from build123d import *

# Parameters (mm, degrees)
SKETCH_1_R               = 5
EXTRUDE_1_DEPTH          = 10
SKETCH_3_R               = 25
SKETCH_3_R_2             = 5
EXTRUDE_4_DEPTH          = 10
EXTRUDE_5_REACH          = 111.952
SKETCH_11_R              = 25
CUT_EXTRUDE_5_DEPTH      = 110.952122557
CUT_EXTRUDE_5_DEPTH_BACK = 110.952122557
SKETCH_13_R              = 18
RIB_2_REACH              = 111.126
SKETCH_14_WALL_W         = 252.93163968
SKETCH_14_WALL_H         = 10
CUT_EXTRUDE_6_DEPTH      = 110.126073878
CUT_EXTRUDE_6_DEPTH_BACK = 5
RIB_3_REACH              = 119.31
SKETCH_18_WALL_W         = 268.526863554
SKETCH_18_WALL_H         = 10


with BuildPart() as part:
    # 草图1 → 凸台-拉伸1 (new body)
    with BuildSketch(Plane(origin=(0, 0, 0), x_dir=(1, 0, 0), z_dir=(0, 1, 0))):
        with BuildLine():
            Line((-50.5, 37.5), (50.5, 37.5))
            ThreePointArc((50.5, 37.5), (58.985281374, 33.985281374), (62.5, 25.5))
            Line((62.5, 25.5), (62.5, -25.5))
            ThreePointArc((62.5, -25.5), (58.985281374, -33.985281374), (50.5, -37.5))
            Line((50.5, -37.5), (-50.5, -37.5))
            ThreePointArc((-50.5, -37.5), (-58.985281374, -33.985281374), (-62.5, -25.5))
            Line((-62.5, -25.5), (-62.5, 25.5))
            ThreePointArc((-62.5, 25.5), (-58.985281374, 33.985281374), (-50.5, 37.5))
        make_face()
        with Locations(Location((50.5, -25.5, 0), (0, 0, 270))):
            Circle(SKETCH_1_R, mode=Mode.SUBTRACT)
        with Locations(Location((50.5, 25.5, 0), (0, 0, 270))):
            Circle(SKETCH_1_R, mode=Mode.SUBTRACT)
        with Locations(Location((-50.5, 25.5, 0), (0, 0, 270))):
            Circle(SKETCH_1_R, mode=Mode.SUBTRACT)
        with Locations(Location((-50.5, -25.5, 0), (0, 0, 270))):
            Circle(SKETCH_1_R, mode=Mode.SUBTRACT)
    extrude(amount=EXTRUDE_1_DEPTH)

    # 草图3 → 凸台-拉伸4 (add)
    with BuildSketch(Plane(origin=(19.955127019, 34.563293868, 0), x_dir=(0, 0, -1), z_dir=(0.500000000000001, 0.866025403784438, 0))):
        with BuildLine():
            Line((-15, -49.126587737), (15, -49.126587737))
            Line((15, -49.126587737), (15, -5.351577729))
            ThreePointArc((15, -5.351577729), (15.986121811, -1.02145071), (18.75, 2.454669769))
            ThreePointArc((18.75, 2.454669769), (22.173981002, 5.666617205), (25.054939633, 9.373412263))
            ThreePointArc((25.054939633, 9.373412263), (28.663169687, 12.676820694), (33.406586177, 13.873412263))
            Line((33.406586177, 13.873412263), (52, 13.873412263))
            ThreePointArc((52, 13.873412263), (64, 25.873412263), (52, 37.873412263))
            Line((52, 37.873412263), (33.406586177, 37.873412263))
            ThreePointArc((33.406586177, 37.873412263), (28.663169687, 39.070003833), (25.054939633, 42.373412263))
            ThreePointArc((25.054939633, 42.373412263), (-20.206795058, 48.047393266), (-18.75, 2.454669769))
            ThreePointArc((-18.75, 2.454669769), (-15.986121811, -1.02145071), (-15, -5.351577729))
            Line((-15, -5.351577729), (-15, -49.126587737))
        make_face()
        with Locations(Location((0, 25.873412263, 0), (0, 0, 90))):
            Circle(SKETCH_3_R, mode=Mode.SUBTRACT)
        with Locations(Location((52, 25.873412263, 0), (0, 0, 90))):
            Circle(SKETCH_3_R_2, mode=Mode.SUBTRACT)
    extrude(amount=-EXTRUDE_4_DEPTH)

    # 凸台-拉伸5: up to this plane
    extrude_5_end = Plane(origin=(50.5, 10, -25.5), z_dir=(0, -1, 0))
    # 草图11 → 凸台-拉伸5 (add, up to the surface)
    with BuildSketch(Plane(origin=(19.955127019, 34.563293868, 0), x_dir=(0.8660254037844382, -0.500000000000001, 0), z_dir=(0.500000000000001, 0.8660254037844382, 0)), mode=Mode.PRIVATE) as extrude_5_sk1:
        with Locations(Location((-25.873412263, 0, 0), (0, 0, 180))):
            Circle(SKETCH_11_R)
    extrude_5_tool1 = split(extrude(extrude_5_sk1.sketch, amount=-EXTRUDE_5_REACH, mode=Mode.PRIVATE), bisect_by=extrude_5_end, keep=Keep.BOTH, mode=Mode.PRIVATE)
    add(extrude_5_tool1.solids().sort_by_distance((-2.451905, 47.5, 0))[0])

    # 草图13 → 切除-拉伸5 (cut, two sides: drawn at the far end of the back side and taken through both)
    with BuildSketch(Plane(origin=(19.955127019, 34.563293868, 0), x_dir=(0, 0, -1), z_dir=(0.500000000000001, 0.866025403784438, 0)).offset(-CUT_EXTRUDE_5_DEPTH_BACK)):
        with Locations(Location((0, 25.873412263, 0), (0, 0, 90))):
            Circle(SKETCH_13_R)
    extrude(amount=CUT_EXTRUDE_5_DEPTH + CUT_EXTRUDE_5_DEPTH_BACK, mode=Mode.SUBTRACT)

    # 草图14 wall → 筋2 (add, up to next)
    with BuildSketch(Plane(origin=(28.349364905, 18.169872981, 0), x_dir=(0.866025403785, -0.499999999999, 0), z_dir=(0.499999999999, 0.866025403785, 0)), mode=Mode.PRIVATE) as rib_2_sk1:
        Rectangle(SKETCH_14_WALL_W, SKETCH_14_WALL_H)
    rib_2_tool1 = extrude(rib_2_sk1.sketch, amount=-RIB_2_REACH, mode=Mode.PRIVATE) - part.part
    add(rib_2_tool1.solids().sort_by_distance((28.349364905, 18.169872981, 0))[0])

    # 草图15 → 切除-拉伸6 (cut, two sides: drawn at the far end of the back side and taken through both)
    with BuildSketch(Plane.XZ.offset(-CUT_EXTRUDE_6_DEPTH_BACK)):
        with BuildLine():
            Line((-41.457999039, 25.5), (41.457999039, 25.5))
            ThreePointArc((41.457999039, 25.5), (44.106339805, 19.106339805), (50.5, 16.457999039))
            Line((50.5, 16.457999039), (50.5, -16.457999039))
            ThreePointArc((50.5, -16.457999039), (44.106339805, -19.106339805), (41.457999039, -25.5))
            Line((41.457999039, -25.5), (-41.457999039, -25.5))
            ThreePointArc((-41.457999039, -25.5), (-44.106339805, -19.106339805), (-50.5, -16.457999039))
            Line((-50.5, -16.457999039), (-50.5, 16.457999039))
            ThreePointArc((-50.5, 16.457999039), (-44.106339805, 19.106339805), (-41.457999039, 25.5))
        make_face()
    extrude(amount=CUT_EXTRUDE_6_DEPTH + CUT_EXTRUDE_6_DEPTH_BACK, mode=Mode.SUBTRACT)

    # 草图18 wall → 筋3 (add, up to next)
    with BuildSketch(Plane(origin=(-14.201905284, 27.148403011, -33.5), x_dir=(-0.423116420047, -0.732859137032, 0.532813269688), z_dir=(-0.266406634844, -0.461429827024, -0.846232840088)), mode=Mode.PRIVATE) as rib_3_sk1:
        Rectangle(SKETCH_18_WALL_W, SKETCH_18_WALL_H)
    rib_3_tool1 = extrude(rib_3_sk1.sketch, amount=-RIB_3_REACH, mode=Mode.PRIVATE) - part.part
    add(rib_3_tool1.solids().sort_by_distance((-14.201905284, 27.148403011, -33.5))[0])


solid = part.part
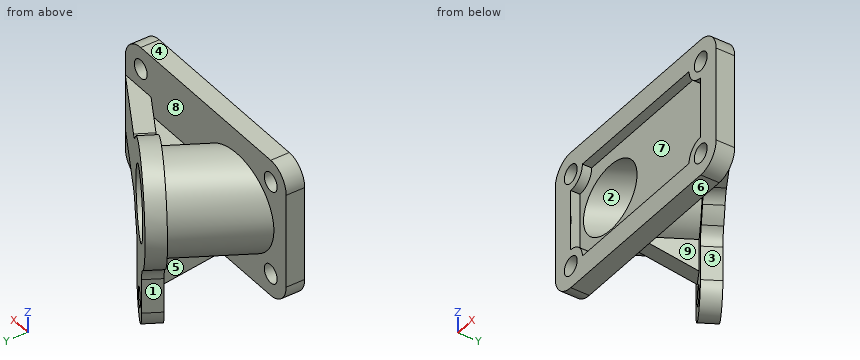
Verification items for the finished model (mm, model axes). Face numbers are marked on the shaded views. A direction names the side the tool comes from. Coordinates: 2 decimals unless noted, no trailing zeros. Write each loop counter-clockwise with the first axis right and the second up, starting at its lowest first coordinate (ties: lowest second). Pieces come first, ordered by that corner, then holes. Notation, with made-up numbers: M 31.5,11 L 35.5,11 A12 ccw 35.5,17 Z; hole C 10,-27 d10. An arc over 180 degrees is marked long. One line per question, with ' | ' between items.
1) Material ranges on L1, parallel to X at y = 6.25, z = 25.5; L2, parallel to X at y = 4, z = 25; L3, parallel to Z at x = -50, y = 4, recorded low to high.
Solutions:
L1: -62.5 to -55.5, -45.5 to 45.5, 55.5 to 62.5 | L2: -62.5 to -55.47, -45.53 to -41.47, 41.47 to 45.53, 55.47 to 62.5 | L3: -37.5 to -30.47, -20.53 to -16.47, 16.47 to 20.53, 30.47 to 37.5
2) Sectioned sample at D-D on z = -12. Record the cut outline in (x, y).
Solutions:
outline: M -62.5,0 L -50.5,0 L -50.5,5 L -42.48,5 L -14.07,54.21 L -26.26,61.25 L -31.26,52.59 L -26.45,49.81 L -49.43,10 L -62.5,10 Z; M -11.5,5 L 50.5,5 L 50.5,0 L 62.5,0 L 62.5,10 L 9.17,40.79 Z; hole M 1.22,10 L 42.5,10 L 11.54,27.87 Z
3) Release check for a two-part mould opening along Y. For the marked faces 1, 2, 3 and 4 record: +Y half, -Y half, draft (parallel to the pull), parting line (faces both ways), or undercut.
Solutions:
face 1: +Y half | face 2: undercut | face 3: undercut | face 4: draft
4) Sectioned sample at B-B on z = -49. Record the cut outline in (x, y).
Solutions:
outline: M -17.84,44.84 L -10.92,40.84 L -5.92,49.5 L -12.84,53.5 Z; M -3.99,36.84 L 2.94,32.84 L 7.94,41.5 L 1.01,45.5 Z
5) Access from +Z, -Z, +X, -X, +Y, -Y to the whole of each face (thin tool, end or side, straight path). Record for the marked faces 5, 6, 7, 8 and 9.
Solutions:
face 5: -Z, -X | face 6: -Z, +X, -X, -Y | face 7: -Y | face 8: none | face 9: -Z
6) Sectioned sample at A-A on z = 8. Record the cut outline in (x, y), then the cut area to 3 significant figures.
Solutions:
outline: M -62.5,0 L -50.5,0 L -50.5,5 L -45.61,5 L -16.42,55.56 L -27.49,61.96 L -32.49,53.3 L -27.96,50.68 L -51.45,10 L -62.5,10 Z; M -8.37,5 L 50.5,5 L 50.5,0 L 62.5,0 L 62.5,10 L 11.51,39.44 Z; hole M 3.25,10 L 42.5,10 L 13.06,27 Z | area: 1,690 mm^2
7) Sectioned sample at C-C on x = 26.5. Record the cut outline in (y, z), then the cut area to 3 significant figures.
Solutions:
outline: M 0,-37.5 L 10,-37.5 L 10,-5 L 19.24,-5 L 19.24,-15 L 30.78,-15 L 30.78,15 L 19.24,15 L 19.24,5 L 10,5 L 10,37.5 L 0,37.5 L 0,25.5 L 5,25.5 L 5,-25.5 L 0,-25.5 Z | area: 934 mm^2
8) Depth check by flat-ended pin: pin 1 Ø4 at (x, z) = (27.5, -19) entering from -Y; pin 2 Ø8.5 at (x, y) = (24, 14.5) entering from -Z; pin 3 Ø11 at (x, y) = (46.5, 19.5) entering from -Z; pin 4 Ø4 at (x, y) = (9.5, 44.5) entering from +Z. Enter the tip coordinate at first touch or a pass-through.
Solutions:
pin 1: y = 5 | pin 2: z = -5 | pin 3: z = -15 | pin 4: through
